Geometry: final body of the model. Coordinates: model frame, mm. Face numbers are marked on the shaded views. A direction names the side the tool comes from. Coordinates: 2 decimals unless noted, no trailing zeros. Write each loop counter-clockwise with the first axis right and the second up, starting at its lowest first coordinate (ties: lowest second). Pieces come first, ordered by that corner, then holes. Notation, with made-up numbers: (10, 60) -> (36, 60) arc R16 ccw to (36, 83) -> close; hole circle Ø4 at (28.25, 9.5). An arc over 180 degrees is marked (long way). One line per item, written item: value.
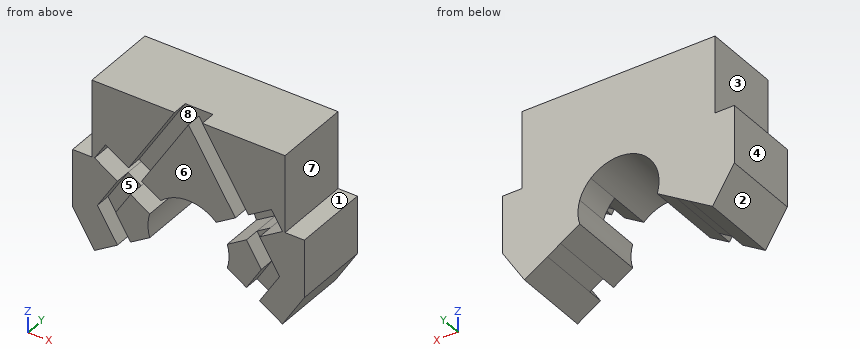
```python
from build123d import *

# Parameters (mm, degrees)
F1_DEPTH = 20
F2_DEPTH = 11
F3_DEPTH = 4


with BuildPart() as f1:
    # F0 (on Front) → F1 (new body)
    with BuildSketch(Plane.XZ):
        with BuildLine():
            ThreePointArc((10.0358588078, 3.0873189), (10.5, 0), (10.0358588078, -3.0873189))
            Line((10.0358588078, -3.0873189), (14.9995515519, -6.1889783681))
            Line((14.9995515519, -6.1889783681), (18.8668544538, 0))
            Line((18.8668544538, 0), (14.9995515519, 6.1889783681))
            Line((14.9995515519, 6.1889783681), (10.0358588078, 3.0873189))
        make_face()
        with BuildLine():
            ThreePointArc((7.1742947809, 7.6667786192), (8.9045050096, 5.5641522744), (10.0358588078, 3.0873189))
            Line((10.0358588078, 3.0873189), (14.9995515519, 6.1889783681))
            Line((14.9995515519, 6.1889783681), (12.1379875251, 10.7684380874))
            Line((12.1379875251, 10.7684380874), (7.1742947809, 7.6667786192))
        make_face()
        Polygon((18.8668544538, 0), (14.9995515519, -6.1889783681), (18.3917439366, -8.308655425), (23.5835680672, 0), (18.3917439366, 8.308655425), (14.9995515519, 6.1889783681), align=None)
        with BuildLine():
            ThreePointArc((-7.1742947809, 7.6667786192), (0, 10.5), (7.1742947809, 7.6667786192))
            Line((7.1742947809, 7.6667786192), (12.1379875251, 10.7684380874))
            Line((12.1379875251, 10.7684380874), (0, 30.1932786368))
            Line((0, 30.1932786368), (-12.1379875251, 10.7684380874))
            Line((-12.1379875251, 10.7684380874), (-7.1742947809, 7.6667786192))
        make_face()
        Polygon((23.5835680672, 0), (18.3917439366, -8.308655425), (24.3280806097, -12.0180902747), (30, -2.9411218284), (30, 12), (25, 12), (25, 32), (3.5877488061, 32), (15.5301799097, 12.8881151443), (21.4665165828, 16.5975499939), (24.3280806097, 12.0180902747), (18.3917439366, 8.308655425), align=None)
        with BuildLine():
            ThreePointArc((-10.0358588078, 3.0873189), (-8.9045050096, 5.5641522744), (-7.1742947809, 7.6667786192))
            Line((-7.1742947809, 7.6667786192), (-12.1379875251, 10.7684380874))
            Line((-12.1379875251, 10.7684380874), (-14.9995515519, 6.1889783681))
            Line((-14.9995515519, 6.1889783681), (-10.0358588078, 3.0873189))
        make_face()
        Polygon((0, 30.1932786368), (12.1379875251, 10.7684380874), (15.5301799097, 12.8881151443), (3.5877488061, 32), (0, 32), (-3.5877488061, 32), (-15.5301799097, 12.8881151443), (-12.1379875251, 10.7684380874), align=None)
        with BuildLine():
            ThreePointArc((-10.0358588078, -3.0873189), (-10.5, 0), (-10.0358588078, 3.0873189))
            Line((-10.0358588078, 3.0873189), (-14.9995515519, 6.1889783681))
            Line((-14.9995515519, 6.1889783681), (-18.8668544538, 0))
            Line((-18.8668544538, 0), (-14.9995515519, -6.1889783681))
            Line((-14.9995515519, -6.1889783681), (-10.0358588078, -3.0873189))
        make_face()
        Polygon((-18.8668544538, 0), (-14.9995515519, 6.1889783681), (-18.3917439366, 8.308655425), (-23.5835680672, 0), (-18.3917439366, -8.308655425), (-14.9995515519, -6.1889783681), align=None)
        Polygon((-21.4665165828, 16.5975499939), (-15.5301799097, 12.8881151443), (-3.5877488061, 32), (-25, 32), (-25, 12), (-30, 12), (-30, -2.9411218284), (-24.3280806097, -12.0180902747), (-18.3917439366, -8.308655425), (-23.5835680672, 0), (-18.3917439366, 8.308655425), (-24.3280806097, 12.0180902747), align=None)
        Polygon((15.5301799097, 12.8881151443), (18.3917439366, 8.308655425), (24.3280806097, 12.0180902747), (21.4665165828, 16.5975499939), align=None)
        Polygon((12.1379875251, 10.7684380874), (14.9995515519, 6.1889783681), (18.3917439366, 8.308655425), (15.5301799097, 12.8881151443), align=None)
        Polygon((-14.9995515519, 6.1889783681), (-12.1379875251, 10.7684380874), (-15.5301799097, 12.8881151443), (-18.3917439366, 8.308655425), align=None)
        Polygon((-18.3917439366, 8.308655425), (-15.5301799097, 12.8881151443), (-21.4665165828, 16.5975499939), (-24.3280806097, 12.0180902747), align=None)
    extrude(amount=-F1_DEPTH)

    # F0 (on Front) → F2 (cut)
    with BuildSketch(Plane.XZ):
        Polygon((15.5301799097, 12.8881151443), (18.3917439366, 8.308655425), (24.3280806097, 12.0180902747), (21.4665165828, 16.5975499939), align=None)
        Polygon((12.1379875251, 10.7684380874), (14.9995515519, 6.1889783681), (18.3917439366, 8.308655425), (15.5301799097, 12.8881151443), align=None)
        with BuildLine():
            ThreePointArc((7.1742947809, 7.6667786192), (8.9045050096, 5.5641522744), (10.0358588078, 3.0873189))
            Line((10.0358588078, 3.0873189), (14.9995515519, 6.1889783681))
            Line((14.9995515519, 6.1889783681), (12.1379875251, 10.7684380874))
            Line((12.1379875251, 10.7684380874), (7.1742947809, 7.6667786192))
        make_face()
        Polygon((-14.9995515519, 6.1889783681), (-12.1379875251, 10.7684380874), (-15.5301799097, 12.8881151443), (-18.3917439366, 8.308655425), align=None)
        with BuildLine():
            ThreePointArc((-10.0358588078, 3.0873189), (-8.9045050096, 5.5641522744), (-7.1742947809, 7.6667786192))
            Line((-7.1742947809, 7.6667786192), (-12.1379875251, 10.7684380874))
            Line((-12.1379875251, 10.7684380874), (-14.9995515519, 6.1889783681))
            Line((-14.9995515519, 6.1889783681), (-10.0358588078, 3.0873189))
        make_face()
        Polygon((-18.3917439366, 8.308655425), (-15.5301799097, 12.8881151443), (-21.4665165828, 16.5975499939), (-24.3280806097, 12.0180902747), align=None)
    extrude(amount=-F2_DEPTH, mode=Mode.SUBTRACT)

    # F0 (on Front) → F3 (cut)
    with BuildSketch(Plane.XZ):
        Polygon((-18.8668544538, 0), (-14.9995515519, 6.1889783681), (-18.3917439366, 8.308655425), (-23.5835680672, 0), (-18.3917439366, -8.308655425), (-14.9995515519, -6.1889783681), align=None)
        Polygon((0, 30.1932786368), (12.1379875251, 10.7684380874), (15.5301799097, 12.8881151443), (3.5877488061, 32), (0, 32), (-3.5877488061, 32), (-15.5301799097, 12.8881151443), (-12.1379875251, 10.7684380874), align=None)
        Polygon((18.8668544538, 0), (14.9995515519, -6.1889783681), (18.3917439366, -8.308655425), (23.5835680672, 0), (18.3917439366, 8.308655425), (14.9995515519, 6.1889783681), align=None)
    extrude(amount=-F3_DEPTH, mode=Mode.SUBTRACT)


solid = f1.part
```
(1) Section A-A (z = -7.5). Return the cut outline in (x, y), then the cut area to 3 significant figures.
Responses:
outline: (-27.15, 0) -> (-18.9, 0) -> (-18.9, 4) -> (-17.1, 4) -> (-17.1, 20) -> (-27.15, 20) -> close; (17.1, 4) -> (18.9, 4) -> (18.9, 0) -> (27.15, 0) -> (27.15, 20) -> (17.1, 20) -> close
area: 388 mm2
(2) Line query: line 1 (X direction, y = 5.25, z = -0.5); line 2 (X direction, y = 9, z = 13.5); line 3 (X direction, y = 4.25, z = 14.5). Output: solid intervals per line, ascending. Write a range as [from, to].
Responses:
line 1: x = [-30, -10.49], [10.49, 30]
line 2: x = [-25, -23.4], [-16.51, 16.51], [23.4, 25]
line 3: x = [-25, -22.78], [-18.11, 18.11], [22.78, 25]
(3) Reachability of the marked faces 1, 2, 3, 4 and 5 from +Z, -Z, +X, -X, +Y, -Y: full face, straight path, thin tool, end or side. Return the list, or none.
Responses:
face 1: +Z, +X, +Y, -Y
face 2: -Z, -X, +Y, -Y
face 3: +Z, -X, +Y, -Y
face 4: +Z, -Z, -X, +Y, -Y
face 5: -Y
(4) Section B-B (y = 8). Return the cut outline in (x, z).
Responses:
outline: (-30, -2.94) -> (-24.33, -12.02) -> (-10.04, -3.09) arc R10.5 cw to (-10.04, 3.09) -> (-24.33, 12.02) -> (-21.47, 16.6) -> (-7.17, 7.67) arc R10.5 cw to (7.17, 7.67) -> (21.47, 16.6) -> (24.33, 12.02) -> (10.04, 3.09) arc R10.5 cw to (10.04, -3.09) -> (24.33, -12.02) -> (30, -2.94) -> (30, 12) -> (25, 12) -> (25, 32) -> (-25, 32) -> (-25, 12) -> (-30, 12) -> close
(5) Section D-D (z = 14). Return the cut outline in (x, y).
Responses:
outline: (-25, 0) -> (-23.09, 0) -> (-23.09, 11) -> (-17.31, 11) -> (-17.31, 0) -> (-14.84, 0) -> (-14.84, 4) -> (-10.12, 4) -> (-10.12, 0) -> (10.12, 0) -> (10.12, 4) -> (14.84, 4) -> (14.84, 0) -> (17.31, 0) -> (17.31, 11) -> (23.09, 11) -> (23.09, 0) -> (25, 0) -> (25, 20) -> (-25, 20) -> close
(6) Pull-direction query (X, two-part tool) for the marked faces 6, 7 and 8; classes: released by +X, released by -X, zero draft, split by the parting line, or undercut.
Responses:
face 6: zero draft
face 7: released by +X
face 8: undercut
(7) Section C-C (x = -16.5). Return the cut outline in (y, z).
Responses:
outline: (0, -3.79) -> (4, -3.79) -> (4, -7.13) -> (20, -7.13) -> (20, 32) -> (0, 32) -> (0, 13.49) -> (11, 13.49) -> (11, 7.13) -> (4, 7.13) -> (4, 3.79) -> (0, 3.79) -> close
(8) First-contact query: pin 1 (1 mm diameter, centred on y = 14.5, z = 22, fed in from -X); pin 2 (6 mm diameter, centred on x = -7, y = 7, fed in from -Z); pin 3 (6 mm diameter, centred on y = 5, z = 19, fed in from +X); pin 4 (7 mm diameter, centred on x = -12, z = 7, fed in from -Y). Flat tips, straight axial feed; report the tip coordinate or a pass-through.
Responses:
pin 1: stops at x = -25
pin 2: stops at z = 7.67
pin 3: stops at x = 25
pin 4: stops at y = 0
